from build123d import *

# Parameters (mm, degrees)
BOSS_EXTRUDE1_DEPTH = 406.4


with BuildPart() as part:
    # Sketch1 → Boss-Extrude1 (new body)
    with BuildSketch(Plane.XY):
        with BuildLine():
            Line((0.79375, 0), (0, 0))
            Line((0, 0), (0, -127))
            ThreePointArc((0, -127), (7.439487758, -144.960512242), (25.4, -152.4))
            Line((25.4, -152.4), (292.1, -152.4))
            ThreePointArc((292.1, -152.4), (310.060512242, -144.960512242), (317.5, -127))
            Line((317.5, -127), (317.5, 0))
            Line((317.5, 0), (316.70625, 0))
            Line((316.70625, 0), (316.70625, -127))
            ThreePointArc((316.70625, -127), (309.499246235, -144.399246235), (292.1, -151.60625))
            Line((292.1, -151.60625), (25.4, -151.60625))
            ThreePointArc((25.4, -151.60625), (8.000753765, -144.399246235), (0.79375, -127))
            Line((0.79375, -127), (0.79375, 0))
        make_face()
        with BuildLine():
            Line((0, -127), (0, 0))
            Line((0, 0), (-0.79375, 0))
            Line((-0.79375, 0), (-0.79375, -127))
            ThreePointArc((-0.79375, -127), (6.87822175, -145.52177825), (25.4, -153.19375))
            Line((25.4, -153.19375), (292.1, -153.19375))
            ThreePointArc((292.1, -153.19375), (310.62177825, -145.52177825), (318.29375, -127))
            Line((318.29375, -127), (318.29375, 0))
            Line((318.29375, 0), (317.5, 0))
            Line((317.5, 0), (317.5, -127))
            ThreePointArc((317.5, -127), (310.060512242, -144.960512242), (292.1, -152.4))
            Line((292.1, -152.4), (25.4, -152.4))
            ThreePointArc((25.4, -152.4), (7.439487758, -144.960512242), (0, -127))
        make_face()
    extrude(amount=BOSS_EXTRUDE1_DEPTH)


solid = part.part
For this review, take the finished solid that the model builds, in its own axes (mm). A direction names the side the tool comes from. Coordinates: 2 decimals unless noted, no trailing zeros. Loops run counter-clockwise (first coordinate to the right, second up) from the corner with the lowest first, then second, coordinate; pieces in that order, holes last. Notation, with made-up numbers: (-30.75, 51) - (6.25, 51) arc R25 cw to (6.25, 71) - close; hole circle Ø2 at (43, 39.5). An arc over 180 degrees is marked (long way). Use a Markdown table: item, result. Add a question column.
Item 1: We need section A-A (y = -36.5). Give the boundary of the cut face in (x, z), and give its area (3 significant figures).
Item 2: For line 1 (X direction, y = -111.5, z = 83.5); line 2 (Y direction, x = 27, z = 239); line 3 (X direction, y = -138.5, z = 79), list the stretches that pass through material, from the lowest coordinate up.
Item 3: Mouldability with a two-part tool opening along X and no side actions: class faces 3 (the face through (157, -153.194, 200)), 4 (the face through (8.193, -144.59, 200.355)), 5 (the face through (316.706, -63, 200)), 6 (the face through (6.68, -145.32, 200.36)) as pulls with the +X half, pulls with the -X half, needs draft (parallel to the pull), parting line crosses it, or undercut.
Item 4: We need section C-C (x = 88.5). Give the boundary of the cut face in (y, z).
Item 5: Insertion check: pin 1 Ø5 at (x, z) = (258, 271) entering from +Y. The pin has a flat end and moves straight along its axis. Give the tip position at first contact, or say it passes through.
Item 6: Tool access review of faces 1 (the face through (161, -151.606, 200)), 2 (the face through (310.42, -145.72, 200.36)): name each direction out of +Z, -Z, +X, -X, +Y, -Y from which nothing blocks a thin tool from reaching the whole face with its end or side.
Item 7: We need section B-B (z = 338.5). Give the boundary of the cut face in (x, y), and give its area (3 significant figures).
Results list:
| question | item | result |
|---|---|---|
| 1 | outline | (-0.79, 0) - (0.79, 0) - (0.79, 406.4) - (-0.79, 406.4) - close; (316.71, 0) - (318.29, 0) - (318.29, 406.4) - (316.71, 406.4) - close |
| 1 | area | 1,290 mm^2 |
| 2 | line 1 | x = -0.79 to 0.79, 316.71 to 318.29 |
| 2 | line 2 | y = -153.19 to -151.61 |
| 2 | line 3 | x = 1.87 to 3.65, 313.85 to 315.63 |
| 3 | face 3 | needs draft |
| 3 | face 4 | undercut |
| 3 | face 5 | undercut |
| 3 | face 6 | pulls with the -X half |
| 4 | outline | (-153.19, 0) - (-151.61, 0) - (-151.61, 406.4) - (-153.19, 406.4) - close |
| 5 | pin 1 | stops at y = -151.61 |
| 6 | face 1 | +Z, -Z, +Y |
| 6 | face 2 | +Z, -Z, +X, -Y |
| 7 | outline | (-0.79, -127) arc R26.19 ccw to (25.4, -153.19) - (292.1, -153.19) arc R26.19 ccw to (318.29, -127) - (318.29, 0) - (316.71, 0) - (316.71, -127) arc R24.61 cw to (292.1, -151.61) - (25.4, -151.61) arc R24.61 cw to (0.79, -127) - (0.79, 0) - (-0.79, 0) - close |
| 7 | area | 953 mm^2 |
